```python
from build123d import *

# Parameters (mm, degrees)
F0_W     = 31.75
F0_H     = 31.75
F1_DEPTH = 10.16
F2_R     = 2.54
F4_R     = 2.2606
F5_DEPTH = 25.4
F6_R     = 3.556
F7_DEPTH = 5.08
F8_R     = 1.143
F9_DEPTH = 25.4


with BuildPart() as f1:
    # F0 (on Top) → F1 (new body)
    with BuildSketch(Plane.XY):
        Rectangle(F0_W, F0_H)
    extrude(amount=F1_DEPTH)

    # F2 (on Front) → F3 (revolve, cut)
    with BuildSketch(Plane.XZ):
        with Locations((5.715, 10.16)):
            Circle(F2_R)
    revolve(axis=Axis((0, 0, 8.061379), (0, 0, -1)), mode=Mode.SUBTRACT)

    # F4 (on face) → F5 (cut)
    with BuildSketch(Plane.XY.offset(10.16)):
        Circle(F4_R)
        with Locations((-8.980256, 8.980256)):
            Circle(F4_R)
        with Locations((8.980256, 8.980256)):
            Circle(F4_R)
        with Locations((-8.980256, -8.980256)):
            Circle(F4_R)
        with Locations((8.980256, -8.980256)):
            Circle(F4_R)
    extrude(amount=-F5_DEPTH, mode=Mode.SUBTRACT)

    # F6 (on face) → F7 (cut)
    with BuildSketch(Plane(origin=(0, 0, 0), x_dir=(1, 0, 0), z_dir=(0, 0, -1))):
        Circle(F6_R)
        with Locations((-8.980256, 8.980256)):
            Circle(F6_R)
        with Locations((8.980256, 8.980256)):
            Circle(F6_R)
        with Locations((-8.980256, -8.980256)):
            Circle(F6_R)
        with Locations((8.980256, -8.980256)):
            Circle(F6_R)
    extrude(amount=-F7_DEPTH, mode=Mode.SUBTRACT)

    # F8 (on face) → F9 (cut)
    with BuildSketch(Plane(origin=(0, 0, 0), x_dir=(1, 0, 0), z_dir=(0, 0, -1))):
        with Locations((-5.715, 0)):
            Circle(F8_R)
    extrude(amount=-F9_DEPTH, mode=Mode.SUBTRACT)


solid = f1.part
```
Here's how the part is built. I have some questions about the finished solid (model axes, mm). A direction names the side the tool comes from. Give positions to 0.01 mm unless a question says otherwise; leave off trailing zeros. Order: outer loops, then holes, each group sorted by start corner. A loop starts at its lowest first (then second) coordinate and runs counter-clockwise, first axis right, second up. Notation, with made-up numbers: (83.25, 45) - (133.25, 45) arc R30 cw to (133.25, 84) - close; hole circle Ø10 at (81, 55.5). An arc over 180 degrees is marked (long way). Answer as a JSON object with one key per item and string values. Group by question number.
Item 1: If we mould it in two halves opening along X, with no side actions, what happens to faces 3 (the cylindrical face through (10.621, 12.135, 2.504)), 4 (the flat face through (0, 15.875, 5)), 5 (the flat face through (-15.875, 0, 5)), 6 (the cylindrical face through (10.196, -7.074, 7.656))? For each: pulls with the +X half, pulls with the -X half, needs draft (parallel to the pull), parting line crosses it, or undercut.
Item 2: Please list where these lines run through material, in increasing order: probe 1 along X at (y, z) = (0, 3.8) (3 decimals); probe 2 along X at (y, z) = (9, 3) (3 decimals); probe 3 along Y at (x, z) = (-9, 10) (3 decimals).
Item 3: Which directions (+Z, -Z, +X, -X, +Y, -Y) give clear straight access to the entire face, cutting with the end or side of a thin tool? Please do faces 1 (the cylindrical face through (-10.77, 7.6, 7.66)), 2 (the flat face through (11.3, 9.7, 5.08)).
Item 4: If we section it at A-A on x = 0: Please give me the cut outline in (y, z) (3 decimals), and give its area (3 significant figures).
Item 5: If we section it at D-D on x = 9.5: Please give me the cut outline in (y, z) (3 decimals).
Item 6: For P1, Ø3.5, axis at x = -8.5, y = -8, coming from the -Z side; P2, Ø2.5, axis at x = -5.715, y = 0, coming from the +Z side, each with a flat end and sliding along its axis, tell me the tip position at first contact or that it passes through.
Item 7: If we section it at C-C on y = 0: Please give me the cut outline in (x, z) (3 decimals).
Item 8: If we section it at B-B on z = 9.5: Please give me the cut outline in (x, y) (1 decimal), and give its area (3 significant figures).
Result set:
{
 "1": {"face 3": "undercut", "face 4": "needs draft", "face 5": "pulls with the -X half", "face 6": "undercut"},
 "2": {"probe 1": "-15.875 to -6.858, -4.572 to -3.556, 3.556 to 15.875", "probe 2": "-15.875 to -12.536, -5.424 to 5.424, 12.536 to 15.875", "probe 3": "-15.875 to -11.241, -6.72 to 6.72, 11.241 to 15.875"},
 "3": {"face 1": "+Z, -Z", "face 2": "-Z"},
 "4": {"outline": "(-15.875, 0) - (-3.556, 0) - (-3.556, 5.08) - (-2.261, 5.08) - (-2.261, 10.16) - (-3.175, 10.16) arc R2.54 cw to (-8.255, 10.16) - (-15.875, 10.16) - close; (2.261, 5.08) - (3.556, 5.08) - (3.556, 0) - (15.875, 0) - (15.875, 10.16) - (8.255, 10.16) arc R2.54 cw to (3.175, 10.16) - (2.261, 10.16) - close", "area": "243 mm²"},
 "5": {"outline": "(-15.875, 0) - (-12.498, 0) - (-12.498, 5.08) - (-11.18, 5.08) - (-11.18, 10.16) - (-15.875, 10.16) - close; (-6.78, 5.08) - (-5.462, 5.08) - (-5.462, 0) - (5.462, 0) - (5.462, 5.08) - (6.78, 5.08) - (6.78, 10.16) - (-6.78, 10.16) - close; (11.18, 5.08) - (12.498, 5.08) - (12.498, 0) - (15.875, 0) - (15.875, 10.16) - (11.18, 10.16) - close"},
 "6": {"P1": "z = 5.08", "P2": "z = 7.95"},
 "7": {"outline": "(-15.875, 0) - (-6.858, 0) - (-6.858, 7.892) arc R2.54 cw to (-8.255, 10.16) - (-15.875, 10.16) - close; (-4.572, 0) - (-3.556, 0) - (-3.556, 5.08) - (-2.261, 5.08) - (-2.261, 10.16) - (-3.175, 10.16) arc R2.54 cw to (-4.572, 7.892) - close; (2.261, 5.08) - (3.556, 5.08) - (3.556, 0) - (15.875, 0) - (15.875, 10.16) - (8.255, 10.16) arc R2.54 cw to (3.175, 10.16) - (2.261, 10.16) - close"},
 "8": {"outline": "(-15.9, -15.9) - (15.9, -15.9) - (15.9, 15.9) - (-15.9, 15.9) - close; circle Ø6.5 at (0, 0); hole circle Ø4.5 at (-9, -9); hole circle Ø4.5 at (-9, 9); hole circle Ø16.3 at (0, 0); hole circle Ø4.5 at (0, 0); hole circle Ø4.5 at (9, -9); hole circle Ø4.5 at (9, 9)", "area": "752 mm²"}
}
